Here's how the part is built. I have some questions about the finished solid (model axes, mm). Round coordinates to 2 decimals unless told otherwise and drop trailing zeros. Loops run counter-clockwise (first coordinate to the right, second up) from the corner with the lowest first, then second, coordinate; pieces in that order, holes last. Notation, with made-up numbers: (-22, 47.25) -> (1, 47.25) arc R38 cw to (1, 86.25) -> close; hole circle Ø9 at (-29.5, 73.5). An arc over 180 degrees is marked (long way). One line per item, written item: value. Start each with the question number.
```python
from build123d import *

# Parameters (mm, degrees)
BOSS_EXTRUDE1_DEPTH = 3
SKETCH2_W           = 10
SKETCH2_H           = 3
SKETCH2_W_2         = 3
SKETCH2_H_2         = 12
CUT_EXTRUDE1_DEPTH  = 10


with BuildPart() as part:
    # Sketch1 → Boss-Extrude1 (new body)
    with BuildSketch(Plane.XY.offset(152)):
        with BuildLine():
            Line((-82, 69.5), (82, 69.5))
            Line((82, 69.5), (82, 44))
            Line((82, 44), (88.6, 44))
            Line((88.6, 44), (88.6, 47))
            Line((88.6, 47), (93.6, 47))
            Line((93.6, 47), (93.6, 44))
            Line((93.6, 44), (98.6, 44))
            Line((98.6, 44), (98.6, 43.377104502))
            ThreePointArc((98.6, 43.377104502), (94.427800977, -13.668492876), (82, -69.5))
            Line((82, -69.5), (-82, -69.5))
            ThreePointArc((-82, -69.5), (-94.427800977, -13.668492876), (-98.6, 43.377104502))
            Line((-98.6, 43.377104502), (-98.6, 44))
            Line((-98.6, 44), (-93.6, 44))
            Line((-93.6, 44), (-93.6, 47))
            Line((-93.6, 47), (-88.6, 47))
            Line((-88.6, 47), (-88.6, 44))
            Line((-88.6, 44), (-82, 44))
            Line((-82, 44), (-82, 69.5))
        make_face()
        with BuildLine():
            Line((-62, -37.134656801), (-62, 37.134656801))
            ThreePointArc((-62, 37.134656801), (-58.87434678, 41.770045043), (-53.405270341, 40.609986811))
            Line((-53.405270341, 40.609986811), (-17.504048439, 3.47533001))
            ThreePointArc((-17.504048439, 3.47533001), (-16.098778099, 0), (-17.504048439, -3.47533001))
            Line((-17.504048439, -3.47533001), (-53.405270341, -40.609986811))
            ThreePointArc((-53.405270341, -40.609986811), (-58.87434678, -41.770045043), (-62, -37.134656801))
        make_face(mode=Mode.SUBTRACT)
        with BuildLine():
            Line((22.39294647, 49.5), (-22.39294647, 49.5))
            ThreePointArc((-22.39294647, 49.5), (-26.996024247, 46.452351141), (-25.987676129, 41.02466999))
            Line((-25.987676129, 41.02466999), (-3.594729659, 17.862383642))
            ThreePointArc((-3.594729659, 17.862383642), (0, 16.337713652), (3.594729659, 17.862383642))
            Line((3.594729659, 17.862383642), (25.987676129, 41.02466999))
            ThreePointArc((25.987676129, 41.02466999), (26.996024247, 46.452351141), (22.39294647, 49.5))
        make_face(mode=Mode.SUBTRACT)
        with BuildLine():
            Line((53.405270341, 40.609986811), (17.504048439, 3.47533001))
            ThreePointArc((17.504048439, 3.47533001), (16.098778099, 0), (17.504048439, -3.47533001))
            Line((17.504048439, -3.47533001), (53.405270341, -40.609986811))
            ThreePointArc((53.405270341, -40.609986811), (58.87434678, -41.770045043), (62, -37.134656801))
            Line((62, -37.134656801), (62, 37.134656801))
            ThreePointArc((62, 37.134656801), (58.87434678, 41.770045043), (53.405270341, 40.609986811))
        make_face(mode=Mode.SUBTRACT)
        with BuildLine():
            Line((-25.987676129, -41.02466999), (-3.594729659, -17.862383642))
            ThreePointArc((-3.594729659, -17.862383642), (0, -16.337713652), (3.594729659, -17.862383642))
            Line((3.594729659, -17.862383642), (25.987676129, -41.02466999))
            ThreePointArc((25.987676129, -41.02466999), (26.996024247, -46.452351141), (22.39294647, -49.5))
            Line((22.39294647, -49.5), (-22.39294647, -49.5))
            ThreePointArc((-22.39294647, -49.5), (-26.996024247, -46.452351141), (-25.987676129, -41.02466999))
        make_face(mode=Mode.SUBTRACT)
    extrude(amount=BOSS_EXTRUDE1_DEPTH)

    # Sketch2 → Cut-Extrude1 (cut)
    with BuildSketch(Plane.XY.offset(155)):
        with Locations((0, 68)):
            Rectangle(SKETCH2_W, SKETCH2_H)
        with Locations((-22, 68)):
            Rectangle(SKETCH2_W, SKETCH2_H)
        with Locations((22, 68)):
            Rectangle(SKETCH2_W, SKETCH2_H)
        with Locations((-44, 68)):
            Rectangle(SKETCH2_W, SKETCH2_H)
        with Locations((44, 68)):
            Rectangle(SKETCH2_W, SKETCH2_H)
        with Locations((-66, 68)):
            Rectangle(SKETCH2_W, SKETCH2_H)
        with Locations((66, 68)):
            Rectangle(SKETCH2_W, SKETCH2_H)
        with Locations((-80.5, 53.5)):
            Rectangle(SKETCH2_W_2, SKETCH2_H_2)
        with Locations((80.5, 53.5)):
            Rectangle(SKETCH2_W_2, SKETCH2_H_2)
        with Locations((-80.5, 31.5)):
            Rectangle(SKETCH2_W_2, SKETCH2_H_2)
        with Locations((-80.5, 9.5)):
            Rectangle(SKETCH2_W_2, SKETCH2_H_2)
        with Locations((-80.5, -12.5)):
            Rectangle(SKETCH2_W_2, SKETCH2_H_2)
        with Locations((-80.5, -34.5)):
            Rectangle(SKETCH2_W_2, SKETCH2_H_2)
        with Locations((-80.5, -56.5)):
            Rectangle(SKETCH2_W_2, SKETCH2_H_2)
        with Locations((80.5, -56.5)):
            Rectangle(SKETCH2_W_2, SKETCH2_H_2)
        with Locations((80.5, -34.5)):
            Rectangle(SKETCH2_W_2, SKETCH2_H_2)
        with Locations((80.5, -12.5)):
            Rectangle(SKETCH2_W_2, SKETCH2_H_2)
        with Locations((80.5, 9.5)):
            Rectangle(SKETCH2_W_2, SKETCH2_H_2)
        with Locations((80.5, 31.5)):
            Rectangle(SKETCH2_W_2, SKETCH2_H_2)
    extrude(amount=-CUT_EXTRUDE1_DEPTH, mode=Mode.SUBTRACT)


solid = part.part
```
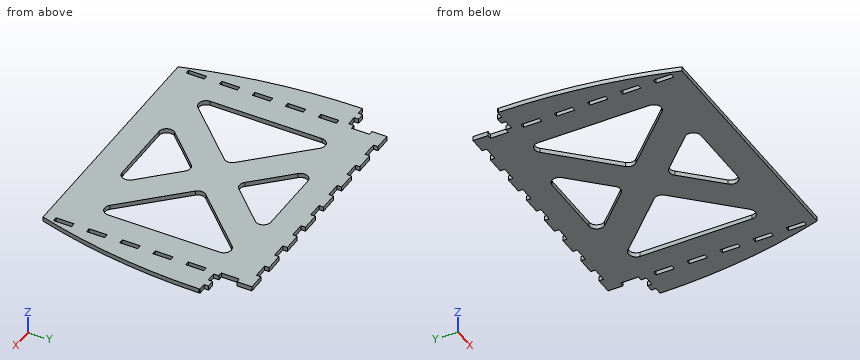
Q1. I want a section at B-B on x = -56. Please give me the cut outline in (y, z).
Q2. I want a section at D-D on y = -10. Please give me the cut outline in (x, z), plus the area to 3 significant figures.
Q3. I want a section at A-A on y = -34.5. Please give me the cut outline in (x, z), plus the area to 3 significant figures.
Q4. Will these pins go through, and if not, where does the flat tip stop? P1, Ø1.5, axis at y = -33.5, z = 153, coming from the -X side; P2, Ø0.9, axis at x = 63.5, z = 153, coming from the +Y side; P3, Ø1.5, axis at x = 86.5, z = 153, coming from the +Y side.
Q5. I want a section at C-C on z = 154. State how many separate pieces and enclosed holes the cut face has, plus the area to 3 significant figures.
Q6. If I drill on line 1 along X through (y, z) = (-0.5, 153.8); line 2 along Y through (x, z) = (-0.5, 154.8); line 3 along Y through (x, z) = (-15, 153.6), over which ranges is the centre line in solid material (lowest first)?
Answers below:
1. outline: (-69.5, 152) -> (-42.03, 152) -> (-42.03, 155) -> (-69.5, 155) -> close; (42.03, 152) -> (69.5, 152) -> (69.5, 155) -> (42.03, 155) -> close
2. outline: (-94.95, 152) -> (-82, 152) -> (-82, 155) -> (-94.95, 155) -> close; (-79, 152) -> (-62, 152) -> (-62, 155) -> (-79, 155) -> close; (-23.81, 152) -> (23.81, 152) -> (23.81, 155) -> (-23.81, 155) -> close; (62, 152) -> (79, 152) -> (79, 155) -> (62, 155) -> close; (82, 152) -> (94.95, 152) -> (94.95, 155) -> (82, 155) -> close
2. area: 323 mm^2
3. outline: (-90.79, 152) -> (-82, 152) -> (-82, 155) -> (-90.79, 155) -> close; (-79, 152) -> (-62, 152) -> (-62, 155) -> (-79, 155) -> close; (-47.5, 152) -> (-19.68, 152) -> (-19.68, 155) -> (-47.5, 155) -> close; (19.68, 152) -> (47.5, 152) -> (47.5, 155) -> (19.68, 155) -> close; (62, 152) -> (79, 152) -> (79, 155) -> (62, 155) -> close; (82, 152) -> (90.79, 152) -> (90.79, 155) -> (82, 155) -> close
3. area: 322 mm^2
4. P1: stops at x = -91.14
4. P2: stops at y = 66.5
4. P3: stops at y = 44
5. separate pieces: 1
5. enclosed holes: 14
5. area: 17,800 mm^2
6. line 1: x = -96.14 to -62, -16.12 to 16.12, 62 to 96.14
6. line 2: y = -69.5 to -49.5, -16.36 to 16.36, 49.5 to 66.5
6. line 3: y = -69.5 to -49.5, -29.66 to 29.66, 49.5 to 69.5
